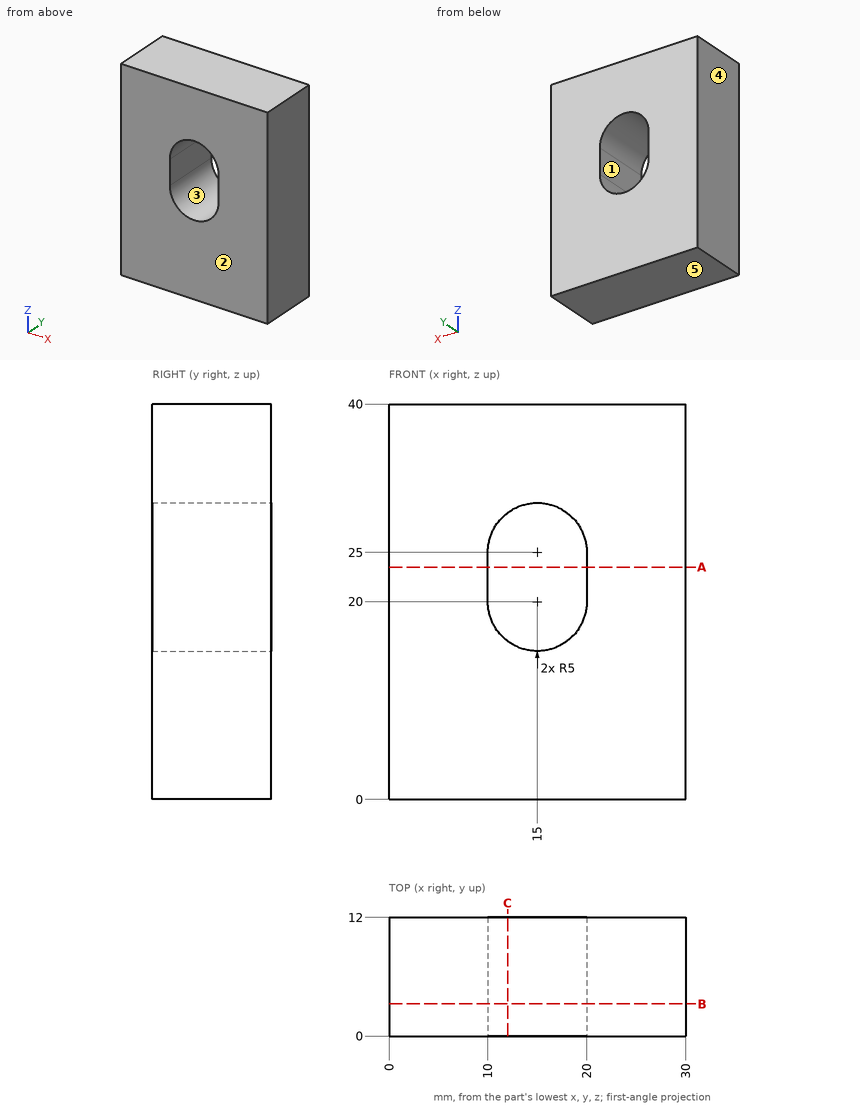
Drawing for the job (mm, zero at the part's lowest x, y, z). A direction names the side the tool comes from. Coordinates: 2 decimals unless noted, no trailing zeros. Order: outer loops, then holes, each group sorted by start corner. A loop starts at its lowest first (then second) coordinate and runs counter-clockwise, first axis right, second up. Notation, with made-up numbers: (-7, 53.25) -> (11, 53.25) arc R16 cw to (11, 60.25) -> close; hole circle Ø2 at (88.5, 1). An arc over 180 degrees is marked (long way). Answer in a Markdown table with one row per item.
1) Mould opens along Z. For the marked faces 3, 4 and 5 say: pulls with the +Z half, pulls with the -Z half, needs draft (parallel to the pull), parting line crosses it, or undercut.
Check values:
| item | result |
|---|---|
| face 3 | undercut |
| face 4 | needs draft |
| face 5 | pulls with the -Z half |
2) Band-saw the part on B-B (y = 3.25). List the corners of the cut face in (x, z).
Check values:
| item | result |
|---|---|
| outline | (0, 0) -> (30, 0) -> (30, 40) -> (0, 40) -> close; hole (10, 20) arc R5 ccw to (20, 20) -> (20, 25) arc R5 ccw to (10, 25) -> close |
3) Which spindle directions (+Z, -Z, +X, -X, +Y, -Y) get a long thin tool onto all of the face, cutting with end or side? Do the marked faces 1 and 2. Say none if no direction does.
Check values:
| item | result |
|---|---|
| face 1 | +Y, -Y |
| face 2 | +Z, -Z, +X, -X, -Y |
4) Band-saw the part on A-A (z = 23.5). List the corners of the cut face in (x, y), and give its area (3 significant figures).
Check values:
| item | result |
|---|---|
| outline | (0, 0) -> (10, 0) -> (10, 12) -> (0, 12) -> close; (20, 0) -> (30, 0) -> (30, 12) -> (20, 12) -> close |
| area | 240 mm2 |
5) Drill centre lines: line 1 (X direction, y = 1.5, z = 25.5); line 2 (X direction, y = 4.5, z = 29.5); line 3 (Z direction, x = 13, y = 6.25). Where is each one in solid material? Low to high.
Check values:
| item | result |
|---|---|
| line 1 | 0 to 10.03, 19.97 to 30 |
| line 2 | 0 to 12.82, 17.18 to 30 |
| line 3 | 0 to 15.42, 29.58 to 40 |
6) Band-saw the part on C-C (x = 12). List the corners of the cut face in (y, z), and give its area (3 significant figures).
Check values:
| item | result |
|---|---|
| outline | (0, 0) -> (12, 0) -> (12, 16) -> (0, 16) -> close; (0, 29) -> (12, 29) -> (12, 40) -> (0, 40) -> close |
| area | 324 mm2 |
